from build123d import *

# Parameters (mm, degrees)
F3_T     = -2.5
F4_R     = 15
F4_R_2   = 12.5
F5_DEPTH = 20
F6_R     = 3


with BuildPart() as f1:
    # F0 (on Right) → F1 (revolve)
    with BuildSketch(Plane.YZ):
        Polygon((0, 0), (0, 30), (-20, 30), (-75, 0), align=None)
    revolve(axis=Axis((0, 0, 15), (0, 0, 1)))

    # F3
    f3_openings = [f1.faces().sort_by_distance(p)[0] for p in [
        (0, 0, 0),
    ]]
    offset(amount=F3_T, openings=f3_openings)

    # F4 (on face) → F5 (join)
    with BuildSketch(Plane.XY.offset(30)):
        Circle(F4_R)
        Circle(F4_R_2, mode=Mode.SUBTRACT)
    extrude(amount=F5_DEPTH)

    # F6
    f6_edges = [f1.edges().sort_by_distance(p)[0] for p in [
        (0, 20, 30),
        (-15, 0, 30),
    ]]
    fillet(f6_edges, radius=F6_R)


solid = f1.part
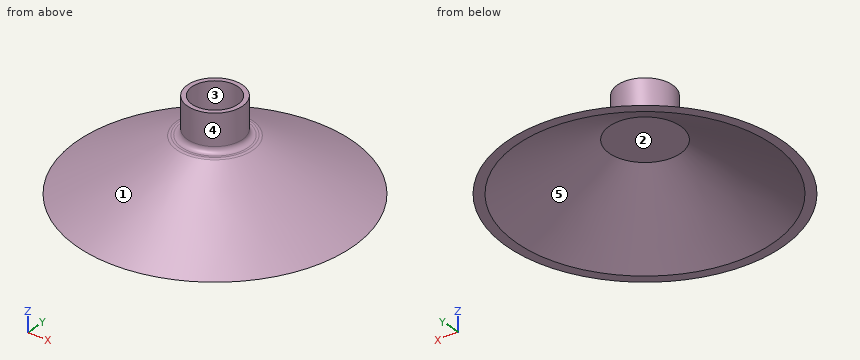
The listing builds one solid part. Answer for the finished solid, in the listing's coordinates (mm). Face numbers are marked on the shaded views. A direction names the side the tool comes from. Give positions to 0.01 mm unless a question says otherwise; leave off trailing zeros. Write each loop counter-clockwise with the first axis right and the second up, starting at its lowest first coordinate (ties: lowest second). Pieces come first, ordered by that corner, then holes.
1) Find the intervals of material crossed by L1, parallel to Y at x = 0, z = 38; L2, parallel to X at y = 20.5, z = 17; L3, parallel to X at y = 11.5, z = 6.5, in increasing order.
2) Section C-C (z = 40.5) is taken. Write down the section's boundary in (x, y).
3) For a pull along Y with two mould halves and no side action, classify the marked faces 3, 4 and 5 as pulls with the +Y half, pulls with the -Y half, needs draft (parallel to the pull), parting line crosses it, or undercut.
4) A tool of negligible diameter and unlimited length cuts with its end or side. For the marked faces 1 and 2, from which of +Z, -Z, +X, -X, +Y, -Y can it reach the whole face along a straight path? Write none if from no direction.
5) Section D-D (z = 22) is taken. Write down the section's boundary in (x, y).
6) Given P1, Ø3, axis at y = 14, z = 30, coming from the -X side; P2, Ø1.5, axis at y = -23.5, z = 14.5, coming from the -X side; P3, Ø1, axis at x = 20.5, y = 1.5, coming from the -Z side, each flat-ended and moving along its own axis, determine where each tip first touches the part or whether it passes through.
7) Section A-A (y = 0) is taken. Write down the section's boundary in (x, z), and give its area (3 significant figures).
Response:
1. L1: y = -15 to -12.5, 12.5 to 15
1. L2: x = -38.74 to -32.72, 32.72 to 38.74
1. L3: x = -62.03 to -56.71, 56.71 to 62.03
2. outline: circle Ø30 at (0, 0); hole circle Ø25 at (0, 0)
3. face 3: undercut
3. face 4: parting line crosses it
3. face 5: undercut
4. face 1: +Z
4. face 2: -Z
5. outline: circle Ø69.33 at (0, 0); hole circle Ø58.89 at (0, 0)
6. P1: stops at x = -18.12
6. P2: stops at x = -43.95
6. P3: stops at z = 26.58
7. outline: (-75, 0) - (-69.78, 0) - (-19.36, 27.5) - (19.36, 27.5) - (69.78, 0) - (75, 0) - (20.67, 29.63) arc R3 ccw to (19.24, 30) - (18, 30) arc R3 cw to (15, 33) - (15, 50) - (12.5, 50) - (12.5, 30) - (-12.5, 30) - (-12.5, 50) - (-15, 50) - (-15, 33) arc R3 cw to (-18, 30) - (-19.24, 30) arc R3 ccw to (-20.67, 29.63) - close
7. area: 502 mm2
